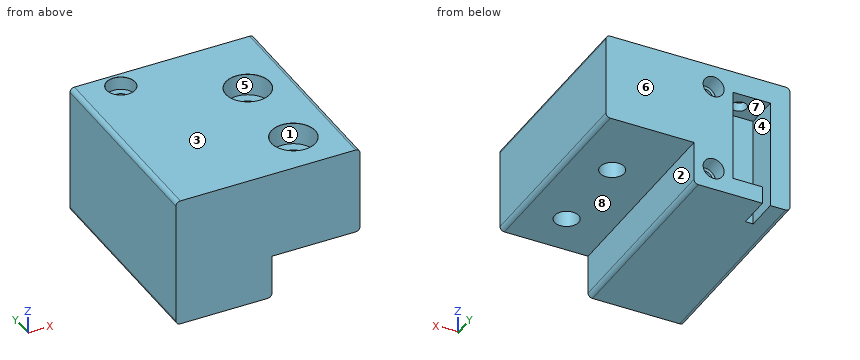
```python
from build123d import *

# Parameters (mm, degrees)
SKETCH1_W                     = 42
SKETCH1_H                     = 20
BOSS_EXTRUDE1_DEPTH           = 40
CBORE_FOR_M5_SHCS1_AT_2_COUNT = 2
CBORE_FOR_M5_SHCS1_AT_2_PITCH = 20
SKETCH5_W                     = 42
SKETCH5_H                     = 20
BOSS_EXTRUDE2_DEPTH           = 6.5
SKETCH12_W                    = 21.9
SKETCH12_H                    = 10
BOSS_EXTRUDE3_DEPTH           = 46.5
CUT_EXTRUDE1_DEPTH            = 7.5
FILLET1_R                     = 1
SKETCH14_R                    = 2.4
CUT_EXTRUDE2_DEPTH            = 3.8
SKETCH15_R                    = 1.7
CUT_EXTRUDE3_DEPTH            = 3


with BuildPart() as part:
    # Sketch1 → Boss-Extrude1 (new body)
    with BuildSketch(Plane(origin=(0, 0, 0), x_dir=(1, 0, 0), z_dir=(0, 1, 0))):
        Rectangle(SKETCH1_W, SKETCH1_H)
    extrude(amount=BOSS_EXTRUDE1_DEPTH)

    # Sketch4 → CBORE for M5 SHCS1 (revolve, cut)
    with BuildSketch(Plane(origin=(11, 30, 10), x_dir=(0, -1, 0), z_dir=(1, 0, 0))):
        Polygon((0, 0), (0, 20), (2.75, 20), (2.75, 5), (5, 5), (5, 0.020977491), (5.025, 0), align=None)
    cbore_for_m5_shcs1 = revolve(axis=Axis((11, 30, 16.35), (0, 0, -1)), mode=Mode.SUBTRACT)

    # CBORE for M5 SHCS1 at 2: CBORE for M5 SHCS1 ×2
    with Locations(*[(0, -i * CBORE_FOR_M5_SHCS1_AT_2_PITCH, 0) for i in range(1, CBORE_FOR_M5_SHCS1_AT_2_COUNT)]):
        add(cbore_for_m5_shcs1, mode=Mode.SUBTRACT)

    # Sketch5 → Boss-Extrude2 (add)
    with BuildSketch(Plane(origin=(0, 40, 0), x_dir=(1, 0, 0), z_dir=(0, 1, 0))):
        Rectangle(SKETCH5_W, SKETCH5_H)
    extrude(amount=BOSS_EXTRUDE2_DEPTH)

    # Sketch12 → Boss-Extrude3 (add)
    with BuildSketch(Plane(origin=(0, 46.5, 0), x_dir=(1, 0, 0), z_dir=(0, 1, 0))):
        with Locations((-10.05, 15)):
            Rectangle(SKETCH12_W, SKETCH12_H)
    extrude(amount=-BOSS_EXTRUDE3_DEPTH)

    # Sketch6 → Cut-Extrude1 (cut)
    with BuildSketch(Plane(origin=(0, 46.5, 0), x_dir=(1, 0, 0), z_dir=(0, 1, 0))):
        Polygon((-16.51, 20), (-16.51, -5), (-8.05, -5), (-8.05, 16), (-14.71, 16), (-14.71, 20), align=None)
    extrude(amount=-CUT_EXTRUDE1_DEPTH, mode=Mode.SUBTRACT)

    # Fillet1
    fillet1_edges = [part.edges().sort_by_distance(p)[0] for p in [
        (0.9, 23.25, -20),
        (-21, 23.25, -20),
        (21, 23.25, -10),
        (21, 23.25, 10),
        (-21, 23.25, 10),
    ]]
    fillet(fillet1_edges, radius=FILLET1_R)

    # Sketch11 → CBORE for M3 SHCS1 (revolve, cut)
    with BuildSketch(Plane(origin=(-11.48, 42.5, 10), x_dir=(0, -1, 0), z_dir=(1, 0, 0))):
        Polygon((0, 0), (0, 6.021463052), (1.7, 5), (1.7, 3), (3.25, 3), (3.25, 0.020977491), (3.275, 0), align=None)
    revolve(axis=Axis((-11.48, 42.5, 16.35), (0, 0, -1)), mode=Mode.SUBTRACT)

    # Sketch14 → Cut-Extrude2 (cut)
    with BuildSketch(Plane(origin=(0, 46.5, 0), x_dir=(1, 0, 0), z_dir=(0, 1, 0))):
        with Locations((-3.575, 15)):
            Circle(SKETCH14_R)
        with Locations((-3.575, -5)):
            Circle(SKETCH14_R)
    extrude(amount=-CUT_EXTRUDE2_DEPTH, mode=Mode.SUBTRACT)

    # Sketch15 → Cut-Extrude3 (cut)
    with BuildSketch(Plane(origin=(0, 42.7, 0), x_dir=(1, 0, 0), z_dir=(0, 1, 0))):
        with Locations((-3.575, 15)):
            Circle(SKETCH15_R)
        with Locations((-3.575, -5)):
            Circle(SKETCH15_R)
    extrude(amount=-CUT_EXTRUDE3_DEPTH, mode=Mode.SUBTRACT)


solid = part.part
```
The model under review builds one solid part; all positions refer to its coordinate system, in mm. Face numbers are marked on the shaded views. A direction names the side the tool comes from. Round coordinates to 2 decimals unless told otherwise and drop trailing zeros. Order: outer loops, then holes, each group sorted by start corner. A loop starts at its lowest first (then second) coordinate and runs counter-clockwise, first axis right, second up. Notation, with made-up numbers: M 46,-3 L 87,-3 A29 ccw 87,36 Z; hole C -28,-0.5 d2. An arc over 180 degrees is marked long. Use a Markdown table: item, result.
1) Wall thickness on line 1 along Y through (x, z) = (11, -5.25); line 2 along X through (y, z) = (44.15, -15) (3 decimals); line 3 along Y through (x, z) = (11, 6.25): over which ranges is each line inside the solid? List them lowest first. Write a range as [from, to].
Report:
| item | result |
|---|---|
| line 1 | [0, 7.25], [12.75, 27.25], [32.75, 46.5] |
| line 2 | [-21, -16.51], [-8.05, -5.975], [-1.175, 0.9] |
| line 3 | [0, 5], [15, 25], [35, 46.5] |
2) Insertion check: pin 1 (6 mm diameter, centred on x = 11, y = 10, fed in from -Z); pin 2 (4.5 mm diameter, centred on x = -3.575, z = -15, fed in from +Y); pin 3 (2 mm diameter, centred on x = 1.5, y = 14.5, fed in from -Z). Each pin has a flat end and moves straight along its axis. Give the tip position at first contact, or say it passes through.
Report:
| item | result |
|---|---|
| pin 1 | z = -10 |
| pin 2 | y = 42.7 |
| pin 3 | z = -19.8 |
3) Consider section D-D (x = -11.48). Write out the cut boundary in (y, z) (3 decimals), then the cut area to 3 significant figures.
Report:
| item | result |
|---|---|
| outline | M 0,-20 L 46.5,-20 L 46.5,-16 L 39,-16 L 39,5 L 40.8,5 L 40.8,7 L 39.25,7 L 39.25,9.979 L 39.225,10 L 0,10 Z; M 44.2,5 L 46.5,5 L 46.5,10 L 45.775,10 L 45.75,9.979 L 45.75,7 L 44.2,7 Z |
| area | 1,210 mm^2 |
4) Consider section A-A (x = 11). Write out the cut boundary in (y, z) (3 decimals).
Report:
| item | result |
|---|---|
| outline | M 0,-10 L 7.25,-10 L 7.25,5 L 5,5 L 5,9.979 L 4.975,10 L 0,10 Z; M 12.75,-10 L 27.25,-10 L 27.25,5 L 25,5 L 25,9.979 L 24.975,10 L 15.025,10 L 15,9.979 L 15,5 L 12.75,5 Z; M 32.75,-10 L 46.5,-10 L 46.5,10 L 35.025,10 L 35,9.979 L 35,5 L 32.75,5 Z |
5) Draft analysis for pull direction X (two halves, no side actions). For the marked faces 1, 2 and 3, state which applies: released by +X, released by -X, zero draft, split by the parting line, or undercut.
Report:
| item | result |
|---|---|
| face 1 | undercut |
| face 2 | released by +X |
| face 3 | zero draft |
6) Consider section C-C (z = -15). Write out the cut boundary in (x, y) (3 decimals).
Report:
| item | result |
|---|---|
| outline | M -21,0 L 0.9,0 L 0.9,46.5 L -1.175,46.5 L -1.175,42.7 L -1.875,42.7 L -1.875,39.7 L -5.275,39.7 L -5.275,42.7 L -5.975,42.7 L -5.975,46.5 L -8.05,46.5 L -8.05,39 L -16.51,39 L -16.51,46.5 L -21,46.5 Z |
7) Consider section B-B (y = 30). Write out the cut boundary in (x, z) (3 decimals).
Report:
| item | result |
|---|---|
| outline | M -21,-19 A1 ccw -20,-20 L -0.1,-20 A1 ccw 0.9,-19 L 0.9,-10 L 8.25,-10 L 8.25,5 L 6,5 L 6,9.979 L 5.975,10 L -20,10 A1 ccw -21,9 Z; M 13.75,-10 L 20,-10 A1 ccw 21,-9 L 21,9 A1 ccw 20,10 L 16.025,10 L 16,9.979 L 16,5 L 13.75,5 Z |
8) Tool access review of the marked faces 4, 5, 6, 7 and 8: name each direction out of +Z, -Z, +X, -X, +Y, -Y from which nothing blocks a thin tool from reaching the whole face with its end or side.
Report:
| item | result |
|---|---|
| face 4 | -Z, +Y |
| face 5 | +Z |
| face 6 | +Z, -Z, +X, -X, +Y |
| face 7 | +Y |
| face 8 | -Z, +X, +Y, -Y |
